For this review, take the finished solid that the model builds, in its own axes (mm). Face numbers are marked on the shaded views. Coordinates: 2 decimals unless noted, no trailing zeros. Loops run counter-clockwise (first coordinate to the right, second up) from the corner with the lowest first, then second, coordinate; pieces in that order, holes last. Notation, with made-up numbers: (69.5, 68) -> (107.5, 68) arc R23 ccw to (107.5, 80) -> close; hole circle Ø6 at (82, 63.5). An arc over 180 degrees is marked (long way). Use a Markdown table: item, result.
from build123d import *

# Parameters (mm, degrees)
SKETCH1_R           = 7.25
BOSS_EXTRUDE1_DEPTH = 0.762
FILLET1_R           = 0.508
SKETCH2_R           = 1.5
BOSS_EXTRUDE2_DEPTH = 2
SKETCH3_R           = 2
BOSS_EXTRUDE3_DEPTH = 2
FILLET2_R           = 1.27


with BuildPart() as part:
    # Sketch1 → Boss-Extrude1 (new body)
    with BuildSketch(Plane.XY):
        with Locations(Location((0, 0, 0), (0, 0, 180))):
            Circle(SKETCH1_R)
    extrude(amount=BOSS_EXTRUDE1_DEPTH)

    # Fillet1
    fillet1_edges = [part.edges().sort_by_distance(p)[0] for p in [
        (7.25, 0, 0),
    ]]
    fillet(fillet1_edges, radius=FILLET1_R)

    # Sketch2 → Boss-Extrude2 (add)
    with BuildSketch(Plane.XY.offset(0.762)):
        Circle(SKETCH2_R)
    extrude(amount=BOSS_EXTRUDE2_DEPTH)

    # Sketch3 → Boss-Extrude3 (add)
    with BuildSketch(Plane.XY.offset(2.762)):
        Circle(SKETCH3_R)
    extrude(amount=BOSS_EXTRUDE3_DEPTH)

    # Fillet2
    fillet2_edges = [part.edges().sort_by_distance(p)[0] for p in [
        (-2, 0, 4.762),
    ]]
    fillet(fillet2_edges, radius=FILLET2_R)


solid = part.part
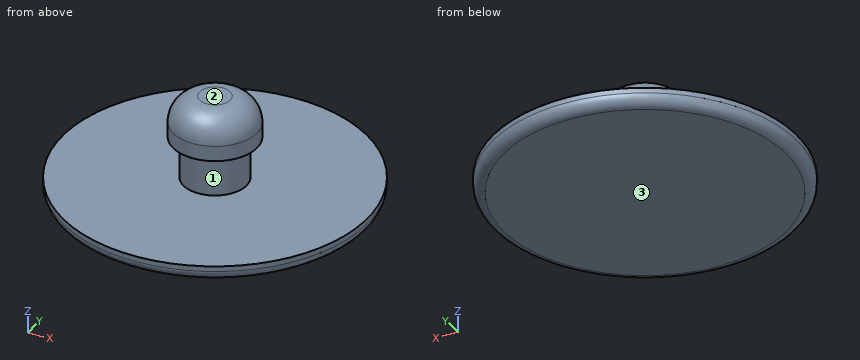
(1) For line 1 along Z through (x, y) = (1.25, -5.5); line 2 along Y through (x, z) = (-0.5, 2.2); line 3 along Y through (x, z) = (-6.5, 0.5), list the stretches that pass through material, from the lowest coordinate up.
Found:
| item | result |
|---|---|
| line 1 | z = 0 to 0.76 |
| line 2 | y = -1.41 to 1.41 |
| line 3 | y = -3.21 to 3.21 |
(2) Mouldability with a two-part tool opening along Z and no side actions: class the marked faces 1, 2 and 3 as pulls with the +Z half, pulls with the -Z half, needs draft (parallel to the pull), parting line crosses it, or undercut.
Found:
| item | result |
|---|---|
| face 1 | undercut |
| face 2 | pulls with the +Z half |
| face 3 | pulls with the -Z half |
(3) For pin 1 Ø5 at (x, y) = (4.5, 4.5) entering from +Z, flat-tipped, find the tip position at first contact; note if it passes through.
Found:
| item | result |
|---|---|
| pin 1 | stops at z = 0.76 |
(4) Take a section at A-A on z = 1.7. Write out the cut boundary in (x, y).
Found:
| item | result |
|---|---|
| outline | circle Ø3 at (0, 0) |
